from build123d import *

# Parameters (mm, degrees)
MAIN_DISC_OUTLINE_R   = 177.8
MAIN_DISC_OUTLINE_W   = 6.35
MAIN_DISC_OUTLINE_H   = 12.7
MAIN_DISC_OUTLINE_W_2 = 12.7
MAIN_DISC_OUTLINE_H_2 = 6.35
MAIN_DISC_DEPTH       = 6.35
SKETCH2_R             = 19.05
SKETCH2_R_2           = 1.8542
SKETCH2_R_3           = 6.35
BEARING_HOLES_DEPTH   = 252.527339468
RACK_HOLES_DEPTH      = 252.527339468


# Read off the part's stored shape, not the designer's step: Main Disc
with BuildPart() as part:
    # Main Disc outline → Main Disc (new body)
    with BuildSketch(Plane(origin=(0, 0, 0), x_dir=(1, 0, 0), z_dir=(0, 1, 0))):
        Circle(MAIN_DISC_OUTLINE_R)
        with Locations((-79.375, -107.95)):
            Rectangle(MAIN_DISC_OUTLINE_W, MAIN_DISC_OUTLINE_H, mode=Mode.SUBTRACT)
        with Locations((-79.375, -82.55)):
            Rectangle(MAIN_DISC_OUTLINE_W, MAIN_DISC_OUTLINE_H, mode=Mode.SUBTRACT)
        with Locations((-82.55, -66.675)):
            Rectangle(MAIN_DISC_OUTLINE_W_2, MAIN_DISC_OUTLINE_H_2, mode=Mode.SUBTRACT)
        with Locations((-31.75, -66.675)):
            Rectangle(MAIN_DISC_OUTLINE_W_2, MAIN_DISC_OUTLINE_H_2, mode=Mode.SUBTRACT)
        with Locations((79.375, -107.95)):
            Rectangle(MAIN_DISC_OUTLINE_W, MAIN_DISC_OUTLINE_H, mode=Mode.SUBTRACT)
        with Locations((31.75, -66.675)):
            Rectangle(MAIN_DISC_OUTLINE_W_2, MAIN_DISC_OUTLINE_H_2, mode=Mode.SUBTRACT)
        with Locations((79.375, -82.55)):
            Rectangle(MAIN_DISC_OUTLINE_W, MAIN_DISC_OUTLINE_H, mode=Mode.SUBTRACT)
        with Locations((82.55, -66.675)):
            Rectangle(MAIN_DISC_OUTLINE_W_2, MAIN_DISC_OUTLINE_H_2, mode=Mode.SUBTRACT)
        with Locations((-82.55, 66.675)):
            Rectangle(MAIN_DISC_OUTLINE_W_2, MAIN_DISC_OUTLINE_H_2, mode=Mode.SUBTRACT)
        with Locations((-79.375, 82.55)):
            Rectangle(MAIN_DISC_OUTLINE_W, MAIN_DISC_OUTLINE_H, mode=Mode.SUBTRACT)
        with Locations((-31.75, 66.675)):
            Rectangle(MAIN_DISC_OUTLINE_W_2, MAIN_DISC_OUTLINE_H_2, mode=Mode.SUBTRACT)
        with Locations((-79.375, 107.95)):
            Rectangle(MAIN_DISC_OUTLINE_W, MAIN_DISC_OUTLINE_H, mode=Mode.SUBTRACT)
        with Locations((-82.55, 123.825)):
            Rectangle(MAIN_DISC_OUTLINE_W_2, MAIN_DISC_OUTLINE_H_2, mode=Mode.SUBTRACT)
        with Locations((-31.75, 123.825)):
            Rectangle(MAIN_DISC_OUTLINE_W_2, MAIN_DISC_OUTLINE_H_2, mode=Mode.SUBTRACT)
        with Locations((31.75, 66.675)):
            Rectangle(MAIN_DISC_OUTLINE_W_2, MAIN_DISC_OUTLINE_H_2, mode=Mode.SUBTRACT)
        with Locations((82.55, 66.675)):
            Rectangle(MAIN_DISC_OUTLINE_W_2, MAIN_DISC_OUTLINE_H_2, mode=Mode.SUBTRACT)
        with Locations((79.375, 82.55)):
            Rectangle(MAIN_DISC_OUTLINE_W, MAIN_DISC_OUTLINE_H, mode=Mode.SUBTRACT)
        with Locations((31.75, 123.825)):
            Rectangle(MAIN_DISC_OUTLINE_W_2, MAIN_DISC_OUTLINE_H_2, mode=Mode.SUBTRACT)
        with Locations((79.375, 107.95)):
            Rectangle(MAIN_DISC_OUTLINE_W, MAIN_DISC_OUTLINE_H, mode=Mode.SUBTRACT)
        with Locations((82.55, 123.825)):
            Rectangle(MAIN_DISC_OUTLINE_W_2, MAIN_DISC_OUTLINE_H_2, mode=Mode.SUBTRACT)
    extrude(amount=MAIN_DISC_DEPTH)

    # Sketch2 → Bearing Holes (cut, through all)
    with BuildSketch(Plane(origin=(0, 6.35, 0), x_dir=(1, 0, 0), z_dir=(0, 1, 0))):
        with Locations(Location((0, 0, 0), (0, 0, 270))):
            Circle(SKETCH2_R)
        with Locations(Location((0, -107.95, 0), (0, 0, 270))):
            Circle(SKETCH2_R_2)
        with Locations(Location((46.020093648, -111.102334226, 0), (0, 0, 270))):
            Circle(SKETCH2_R_3)
        with Locations(Location((107.95, 0, 0), (0, 0, 270))):
            Circle(SKETCH2_R_2)
        with Locations(Location((0, 107.95, 0), (0, 0, 270))):
            Circle(SKETCH2_R_2)
        with Locations(Location((-107.95, 0, 0), (0, 0, 270))):
            Circle(SKETCH2_R_2)
    extrude(amount=-BEARING_HOLES_DEPTH, mode=Mode.SUBTRACT)

    # Sketch3 → Rack Holes (cut, through all)
    with BuildSketch(Plane(origin=(0, 6.35, 0), x_dir=(1, 0, 0), z_dir=(0, 1, 0))):
        with BuildLine():
            ThreePointArc((-170.495993222, -11.296428481), (-170.496985984, -11.235760757), (-170.499963206, -11.175157998))
            Line((-170.499963206, -11.175157998), (-172.350193222, -11.296428481))
            ThreePointArc((-172.350193222, -11.296428481), (-172.4083456, -10.371150737), (-172.461530575, -9.445574182))
            ThreePointArc((-172.461530575, -9.445574182), (-173.621337572, -12.646335766), (-170.495993222, -11.296428481))
        make_face()
        with BuildLine():
            Line((-172.350193222, -11.296428481), (-170.499963206, -11.175157998))
            ThreePointArc((-170.499963206, -11.175157998), (-171.123897186, -9.905653275), (-172.461530575, -9.445574182))
            ThreePointArc((-172.461530575, -9.445574182), (-172.4083456, -10.371150737), (-172.350193222, -11.296428481))
        make_face()
        with BuildLine():
            ThreePointArc((-123.435544137, 120.813347125), (-122.126506883, 120.277289924), (-120.820365853, 120.820365853))
            Line((-120.820365853, 120.820365853), (-122.131483247, 122.131483247))
            ThreePointArc((-122.131483247, 122.131483247), (-122.785282527, 121.474165133), (-123.435544137, 120.813347125))
        make_face()
        with BuildLine():
            Line((-122.131483247, 122.131483247), (-120.820365853, 120.820365853))
            ThreePointArc((-120.820365853, 120.820365853), (-120.418425817, 121.421911626), (-120.277283247, 122.131483247))
            ThreePointArc((-120.277283247, 122.131483247), (-120.416527615, 122.836454751), (-120.813347125, 123.435544137))
            ThreePointArc((-120.813347125, 123.435544137), (-121.474165133, 122.785282527), (-122.131483247, 122.131483247))
        make_face()
        with BuildLine():
            ThreePointArc((-120.813347125, 123.435544137), (-123.44260064, 123.44260064), (-123.435544137, 120.813347125))
            ThreePointArc((-123.435544137, 120.813347125), (-122.785282527, 121.474165133), (-122.131483247, 122.131483247))
            ThreePointArc((-122.131483247, 122.131483247), (-121.474165133, 122.785282527), (-120.813347125, 123.435544137))
        make_face()
        with BuildLine():
            ThreePointArc((9.445574182, 172.461530575), (9.905653275, 171.123897186), (11.175157998, 170.499963206))
            Line((11.175157998, 170.499963206), (11.296428481, 172.350193222))
            ThreePointArc((11.296428481, 172.350193222), (10.371150737, 172.4083456), (9.445574182, 172.461530575))
        make_face()
        with BuildLine():
            Line((11.296428481, 172.350193222), (11.175157998, 170.499963206))
            ThreePointArc((11.175157998, 170.499963206), (12.563945327, 170.996879258), (13.150628481, 172.350193222))
            ThreePointArc((13.150628481, 172.350193222), (11.352122286, 174.203556608), (9.445574182, 172.461530575))
            ThreePointArc((9.445574182, 172.461530575), (10.371150737, 172.4083456), (11.296428481, 172.350193222))
        make_face()
    extrude(amount=-RACK_HOLES_DEPTH, mode=Mode.SUBTRACT)


solid = part.part
Read the model definition and answer for the solid it produces. Units are mm, in the model's axes. Round coordinates to 2 decimals unless told otherwise and drop trailing zeros. Write each loop counter-clockwise with the first axis right and the second up, starting at its lowest first coordinate (ties: lowest second). Pieces come first, ordered by that corner, then holes.
Q1. Find section A-A on x = -14. Determine the outline of the cut face in (y, z), and give its area (3 significant figures).
Values:
outline: (0, -177.25) - (6.35, -177.25) - (6.35, -12.92) - (0, -12.92) - close; (0, 12.92) - (6.35, 12.92) - (6.35, 177.25) - (0, 177.25) - close
area: 2,090 mm2
Q2. The mould has two halves that part along X. Classify faces 1 (the face through (-11.59, 3.22, -15.12)), 2 (the face through (-2, 0, 37)), 3 (the face through (169.59, 3.13, -53.41)): released by +X, released by -X, zero draft, split by the parting line, or undercut.
Values:
face 1: undercut
face 2: zero draft
face 3: split by the parting line
Q3. Straight lines are drawn through the part: line 1 (X direction, y = 2, z = 0); line 2 (X direction, y = 4, z = -107.95); line 3 (X direction, y = 5.25, z = -110). For each, find the intervals that lie inside material, in ascending order.
Values:
line 1: x = -177.8 to -109.8, -106.1 to -19.05, 19.05 to 106.1, 109.8 to 177.8
line 2: x = -141.28 to -82.55, -76.2 to -1.85, 1.85 to 76.2, 82.55 to 141.28
line 3: x = -139.69 to -82.55, -76.2 to 76.2, 82.55 to 139.69
Q4. Find section B-B on y = 5. State how many separate pieces and enclosed holes the cut face has, and give its area (3 significant figures).
Values:
separate pieces: 1
enclosed holes: 29
area: 96,400 mm2
Q5. Find section C-C on z = 143. Determine the outline of the cut face in (x, y).
Values:
outline: (-105.66, 0) - (105.66, 0) - (105.66, 6.35) - (-105.66, 6.35) - close
Q6. Find section D-D on z = 34.5. Determine the outline of the cut face in (x, y), and give its area (3 significant figures).
Values:
outline: (-174.42, 0) - (174.42, 0) - (174.42, 6.35) - (-174.42, 6.35) - close
area: 2,220 mm2
Q7. Flat-ended cylindrical pins translate along their axes: P1, Ø3, axis at x = -107, y = 4, coming from the +Z side; P2, Ø1.5, axis at y = 4.5, z = -137, coming from the +X side; P3, Ø3, axis at y = 1.5, z = -123.5, coming from the -X side. Find the tip coordinate at first contact, or state that the pin passes through.
Values:
P1: stops at z = 143.12
P2: stops at x = 114.23
P3: stops at x = -129.34
